Verification items for the finished model (mm, model axes). A direction names the side the tool comes from. Coordinates: 2 decimals unless noted, no trailing zeros. Write each loop counter-clockwise with the first axis right and the second up, starting at its lowest first coordinate (ties: lowest second). Pieces come first, ordered by that corner, then holes. Notation, with made-up numbers: (55, 54.5) - (92, 54.5) arc R31 cw to (92, 90.5) - close; hole circle Ø1 at (-14.5, 64). An arc over 180 degrees is marked (long way). Answer as CSV lines item,"result". Start each with the question number.
```python
from build123d import *

# Parameters (mm, degrees)
F0_W     = 254
F0_H     = 127
F1_DEPTH = 25.4
F0_W_2   = 25.4
F0_H_2   = 12.7
F2_DEPTH = 12.7
F3_W     = 304.8
F3_H     = 12.7
F4_DEPTH = 25.4


with BuildPart() as f1:
    # F0 (on Top) → F1 (new body)
    with BuildSketch(Plane.XY):
        with Locations((-2.477834, -50.816161)):
            Rectangle(F0_W, F0_H)
    extrude(amount=F1_DEPTH)

    # F0 (on Top) → F2 (join)
    with BuildSketch(Plane.XY):
        with Locations((-142.177834, 19.033839)):
            Rectangle(F0_W_2, F0_H_2)
        with Locations((-2.477834, 19.033839)):
            Rectangle(F0_W, F0_H_2)
        with Locations((-142.177834, -50.816161)):
            Rectangle(F0_W_2, F0_H)
        with Locations((137.222166, 19.033839)):
            Rectangle(F0_W_2, F0_H_2)
        with Locations((-142.177834, -120.666161)):
            Rectangle(F0_W_2, F0_H_2)
        with Locations((137.222166, -50.816161)):
            Rectangle(F0_W_2, F0_H)
        with Locations((-2.477834, -120.666161)):
            Rectangle(F0_W, F0_H_2)
        with Locations((137.222166, -120.666161)):
            Rectangle(F0_W_2, F0_H_2)
    extrude(amount=F2_DEPTH)

    # F3 (on face) → F4 (cut)
    with BuildSketch(Plane(origin=(0, 0, 0), x_dir=(1, 0, 0), z_dir=(0, 0, -1))):
        with Locations((-2.477834, 120.666161)):
            Rectangle(F3_W, F3_H)
        with Locations((-2.477834, -19.033839)):
            Rectangle(F3_W, F3_H)
    extrude(amount=-F4_DEPTH, mode=Mode.SUBTRACT)


solid = f1.part
```
1. Cross-section at B-B (z = 22). Record the cut outline in (x, y), and give its area (3 significant figures).
2. Scan lines: line 1 along X through (y, z) = (-91.5, 24.75); line 2 along Z through (x, y) = (129, -22.5). Record each from-to range of solid material in increasing order. Write a range as from..to.
3. Cross-section at A-A (y = -73.5). Record the cut outline in (x, z).
4. Depth check by flat-ended pin: P1, Ø6.5, axis at y = -73, z = 18, coming from the -X side; P2, Ø20.5, axis at x = -145.5, y = -75.5, coming from the +Z side; P3, Ø1.5, axis at y = -17.5, z = 22, coming from the +X side; P4, Ø10, axis at y = -68, z = 17.5, coming from the +X side. Enter the tip coordinate at first touch or a pass-through.
5. Access from +Z, -Z, +X, -X, +Y, -Y to the whole of each face (thin tool, end or side, straight path). Record for faces 1 (the face through (-5, -50, 0)), 2 (the face through (-129.478, -52, 19)), 3 (the face through (137, -50, 12.7)).
Completed:
1,outline,"(-129.48, -114.32) - (124.52, -114.32) - (124.52, 12.68) - (-129.48, 12.68) - close"
1,area,"32,300 mm2"
2,line 1,"x = -129.48..124.52"
2,line 2,"z = 0..12.7"
3,outline,"(-154.88, 0) - (149.92, 0) - (149.92, 12.7) - (124.52, 12.7) - (124.52, 25.4) - (-129.48, 25.4) - (-129.48, 12.7) - (-154.88, 12.7) - close"
4,P1,"stops at x = -129.48"
4,P2,"stops at z = 12.7"
4,P3,"stops at x = 124.52"
4,P4,"stops at x = 149.92"
5,face 1,"-Z, +X, -X, +Y, -Y"
5,face 2,"+Z, -X, +Y, -Y"
5,face 3,"+Z, +X, +Y, -Y"
